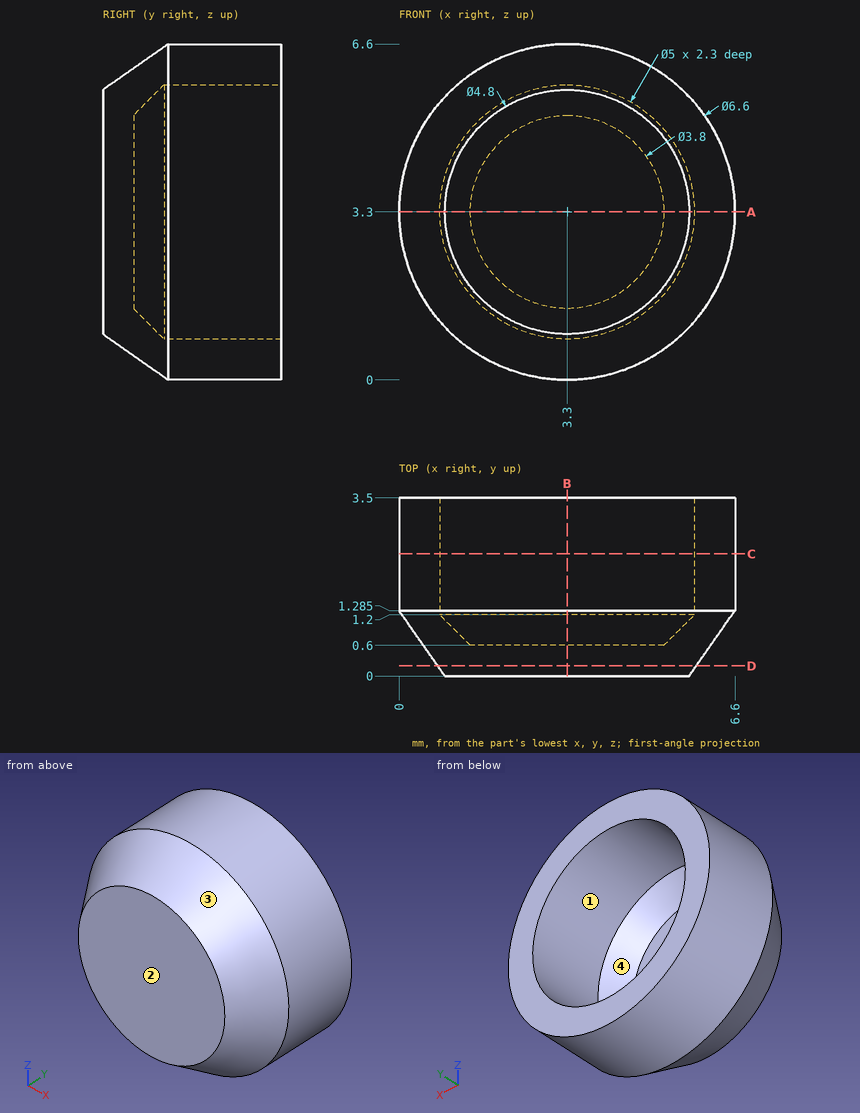
Design review of the part shown in the three views and the two pictorial views. Dimensions are in mm from the part's minimum x, y and z. Round coordinates to 2 decimals unless told otherwise and drop trailing zeros. Write each loop counter-clockwise with the first axis right and the second up, starting at its lowest first coordinate (ties: lowest second). Pieces come first, ordered by that corner, then holes. Notation, with made-up numbers: (18.25, 5.5) -> (57.25, 5.5) arc R23 ccw to (57.25, 33.5) -> close; hole circle Ø4 at (-6, -29). An arc over 180 degrees is marked (long way). One line per question, with ' | ' between items. Start each with the question number.
1) Add section A-A (z = 3.3). Write out the cut boundary in (x, y) (1 decimal).
2) Add section C-C (y = 2.4). Write out the cut boundary in (x, z), and give its area (3 significant figures).
3) Add section D-D (y = 0.2). Write out the cut boundary in (x, z), and give its area (3 significant figures).
4) For pin 1 Ø2 at (y, z) = (1.5, 1.5) entering from +X; pin 2 Ø1.5 at (y, z) = (1.5, 1.5) entering from -X, all flat-tipped, find the tip position at first contact; note any pin that passes through.
5) Mouldability with a two-part tool opening along X and no side actions: class the marked faces 1, 2, 3 and 4 as +X half, -X half, draft (parallel to the pull), parting line (faces both ways), or undercut.
6) Wall thickness on line 1 along X through (y, z) = (1.85, 3.3); line 2 along Z through (x, y) = (1.75, 2.4) (1 decimal); line 3 along X through (y, z) = (1.05, 3): over which ranges is each line inside the solid? List them lowest first.
7) Add section B-B (x = 3.3). Write out the cut boundary in (y, z) (1 decimal).
Reported:
1) outline: (0, 1.3) -> (0.9, 0) -> (5.7, 0) -> (6.6, 1.3) -> (6.6, 3.5) -> (5.8, 3.5) -> (5.8, 1.2) -> (5.2, 0.6) -> (1.4, 0.6) -> (0.8, 1.2) -> (0.8, 3.5) -> (0, 3.5) -> close
2) outline: circle Ø6.6 at (3.3, 3.3); hole circle Ø5 at (3.3, 3.3) | area: 14.6 mm²
3) outline: circle Ø5.08 at (3.3, 3.3) | area: 20.3 mm²
4) pin 1: stops at x = 6.5 | pin 2: stops at x = 0.17
5) face 1: undercut | face 2: draft | face 3: parting line | face 4: undercut
6) line 1: x = 0 to 0.8, 5.8 to 6.6 | line 2: z = 0.4 to 1.3, 5.3 to 6.2 | line 3: x = 0.18 to 0.97, 5.63 to 6.42
7) outline: (0, 0.9) -> (1.3, 0) -> (3.5, 0) -> (3.5, 0.8) -> (1.2, 0.8) -> (0.6, 1.4) -> (0.6, 5.2) -> (1.2, 5.8) -> (3.5, 5.8) -> (3.5, 6.6) -> (1.3, 6.6) -> (0, 5.7) -> close
